Can you work these out from the model? Positions are in its coordinate system, mm. Face numbers are marked on the shaded views. Round coordinates to 2 decimals unless told otherwise and drop trailing zeros. Order: outer loops, then holes, each group sorted by start corner. A loop starts at its lowest first (then second) coordinate and runs counter-clockwise, first axis right, second up. Notation, with made-up numbers: M 81,82 L 123,82 A25 cw 123,118 Z; hole C -10.75,10.25 d11. An arc over 180 degrees is marked long. Answer as a JSON object with one key per item and string values. Group by question number.
Autodesk Inventor part; units mm, degrees
ref_plane "YZ Plane" through (0, 0, 0) normal (1, 0, 0) x (0, 1, 0)
ref_plane "XZ Plane" through (0, 0, 0) normal (0, 1, 0) x (-1, 0, 0)
ref_plane "XY Plane" through (0, 0, 0) normal (0, 0, 1) x (1, 0, 0)
sketch "Sketch1" plane through (0, 0, 0) normal (0, 1, 0) x (-1, 0, 0)
  line L0 (25.4, 12.7) -> (-25.4, 12.7)
  line L1 (-25.4, 12.7) -> (-25.4, -12.7)
  line L2 (-25.4, -12.7) -> (25.4, -12.7)
  line L3 (25.4, -12.7) -> (25.4, 12.7)
  line L4 (25.4, 12.7) -> (-25.4, -12.7) construction
  line L5 (-25.4, 12.7) -> (25.4, -12.7) construction
  point P0 (0, 0)
  dimension "d0" = 25.4
  dimension "d1" = 50.8
extrude "Extrusion1" add sketch "Sketch1" against normal blind 38.1
sketch "Sketch2" plane through (-25.4, 0, 12.7) normal (0, 0, 1) x (1, 0, 0)
  line L0 (50.8, -38.1) -> (0, -38.1)
  circle A0 centre (25.4, -38.1) radius 6.35
  point P0 (25.4, 0)
  dimension "d4" = 12.7
extrude "Extrusion2" cut sketch "Sketch2" against normal through all
properties part number "StandAloneLift"
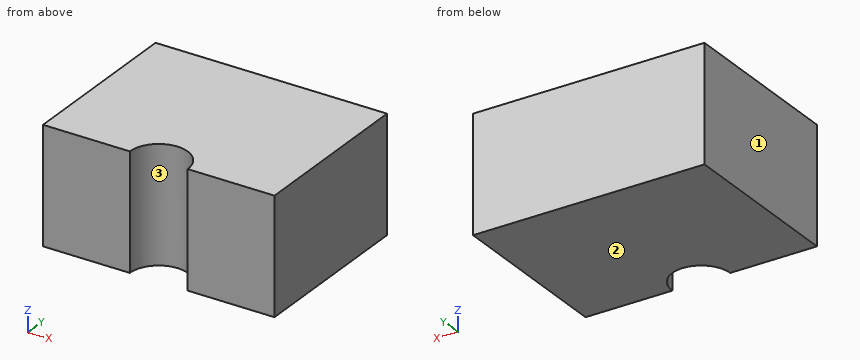
Item 1: I need wall thicknesses on line 1 (Y direction, x = -1.5, z = -1.75); line 2 (Y direction, x = -5, z = -8). Which ranges of each line are inside material? Lowest first, please.
Item 2: Suppose I cut it at B-B, the plane z = -2.75. Write out the boundary of the cut face in (x, y), and give its area (3 significant figures).
Item 3: Suppose I cut it at C-C, the plane x = 0. Write out the boundary of the cut face in (y, z).
Item 4: If we mould it in two halves opening along X, with no side actions, what happens to the marked faces 1, 2 and 3? For each: +X half, -X half, draft (parallel to the pull), parting line (faces both ways), or undercut.
Item 5: Suppose I cut it at A-A, the plane y = -36. Write out the boundary of the cut face in (x, z).
Item 6: I'm going to push a flat-ended pin straight in: pin 1 Ø6 at (x, z) = (-11.5, -2.5) entering from +Y. Where does the tip first touch, or does it pass through?
Computed:
{
 "1": {"line 1": "y = -31.93 to 0", "line 2": "y = -34.19 to 0"},
 "2": {"outline": "M -25.4,-38.1 L -6.35,-38.1 A6.35 cw 6.35,-38.1 L 25.4,-38.1 L 25.4,0 L -25.4,0 Z", "area": "1,870 mm^2"},
 "3": {"outline": "M -31.75,-12.7 L 0,-12.7 L 0,12.7 L -31.75,12.7 Z"},
 "4": {"face 1": "-X half", "face 2": "draft", "face 3": "undercut"},
 "5": {"outline": "M -25.4,-12.7 L -5.99,-12.7 L -5.99,12.7 L -25.4,12.7 Z; M 5.99,-12.7 L 25.4,-12.7 L 25.4,12.7 L 5.99,12.7 Z"},
 "6": {"pin 1": "stops at y = 0"}
}
